Verification items for the finished model (mm, model axes). A direction names the side the tool comes from. Round coordinates to 2 decimals unless told otherwise and drop trailing zeros. Order: outer loops, then holes, each group sorted by start corner. A loop starts at its lowest first (then second) coordinate and runs counter-clockwise, first axis right, second up. Notation, with made-up numbers: (46, 25) -> (59, 25) arc R14 cw to (59, 42) -> close; hole circle Ø11 at (8, 17). An arc over 180 degrees is marked (long way). Return JSON: item names as keys, results as strings. Group by question number.
1) Tool access check on faces 1 (the cylindrical face through (0.867, -3.905, 0.159)), 2 (the cylindrical face through (4.619, -1.915, 13.795)). Record the directions out of +Z, -Z, +X, -X, +Y, -Y that give a thin tool (end or side, any length) a straight path to the whole face; none if there is none.
2) Section check A-A on z = 70.5. Enter the section's corners in (x, y), plus the area to 3 significant figures.
3) Depth check by flat-ended pin: pin 1 (2 mm diameter, centred on y = 3.5, z = 51.5, fed in from -X); pin 2 (5 mm diameter, centred on x = -3, z = 58, fed in from +Y); pin 3 (6 mm diameter, centred on y = -3.5, z = 72, fed in from +X). Enter the tip coordinate at first touch or a pass-through.
4) Draft check along Z on faces 3 (the cylindrical face through (4.619, -1.915, 46.394)), 4 (the cylindrical face through (0.867, -3.905, 27.893)), 5 (the flat face through (0, 0, 135)). Enter one of: pulls with the +Z half, pulls with the -Z half, needs draft (parallel to the pull), parting line crosses it, or undercut.
5) Scan lines: L1, parallel to Z at x = 4, y = -2.25 (3 decimals); L2, parallel to X at y = -0.5, z = 119; L3, parallel to Y at x = 0.25, z = 42. Record each from-to range of solid material in increasing order.
```python
from build123d import *

# Parameters (mm, degrees)
SKETCH1_R           = 5
BOSS_EXTRUDE1_DEPTH = 135
SKETCH2_W           = 1
SKETCH2_H           = 0.8
BOSS_EXTRUDE2_START = 5
SKETCH3_R           = 5
BOSS_EXTRUDE2_DEPTH = 5
SKETCH4_R           = 5
SKETCH4_R_2         = 4
CUT_EXTRUDE1_DEPTH  = 0.8
SKETCH5_R           = 5
SKETCH5_R_2         = 4
CUT_EXTRUDE2_DEPTH  = 1


with BuildPart() as part:
    # Sketch1 → Boss-Extrude1 (new body)
    with BuildSketch(Plane.XY):
        Circle(SKETCH1_R)
    extrude(amount=BOSS_EXTRUDE1_DEPTH)

    # Sketch2 → Cut-Revolve1 (revolve, cut)
    with BuildSketch(Plane(origin=(0, 0, 0), x_dir=(1, 0, 0), z_dir=(0, 1, 0))):
        with Locations((-4.5, -65.3)):
            Rectangle(SKETCH2_W, SKETCH2_H)
        with Locations((-4.5, -93.4)):
            Rectangle(SKETCH2_W, SKETCH2_H)
    revolve(axis=Axis((0, 0, 6.050553304), (0, 0, 1)), mode=Mode.SUBTRACT)

    # Sketch3 → Boss-Extrude2 (add)
    with BuildSketch(Plane(origin=(0, 0, 0), x_dir=(-1, 0, 0), z_dir=(0, 0, -1)).offset(BOSS_EXTRUDE2_START)):
        Circle(SKETCH3_R)
    extrude(amount=-BOSS_EXTRUDE2_DEPTH)

    # Sketch4 → Cut-Extrude1 (cut)
    with BuildSketch(Plane(origin=(-672.545878218, -100.484437541, -0.235), x_dir=(-0.3247374432468007, 0.945804204343336, 0), z_dir=(0, 0, -1))):
        with Locations(Location((-123.362225461, 668.727778566, 0), (0, 0, 288.949668831))):
            Circle(SKETCH4_R)
        with Locations(Location((-123.362225461, 668.727778566, 0), (0, 0, 288.949668831))):
            Circle(SKETCH4_R_2, mode=Mode.SUBTRACT)
    extrude(amount=-CUT_EXTRUDE1_DEPTH, mode=Mode.SUBTRACT)

    # Sketch5 → Cut-Extrude2 (cut)
    with BuildSketch(Plane(origin=(-672.545878218, -100.484437541, 27.4), x_dir=(-0.3247374432468007, 0.945804204343336, 0), z_dir=(0, 0, -1))):
        with Locations(Location((-123.362225461, 668.727778566, 0), (0, 0, 288.949668831))):
            Circle(SKETCH5_R)
        with Locations(Location((-123.362225461, 668.727778566, 0), (0, 0, 288.949668831))):
            Circle(SKETCH5_R_2, mode=Mode.SUBTRACT)
    extrude(amount=-CUT_EXTRUDE2_DEPTH, mode=Mode.SUBTRACT)


solid = part.part
```
Check result:
{
 "1": {"face 1": "none", "face 2": "+Z, -Z"},
 "2": {"outline": "circle Ø10 at (0, 0)", "area": "78.5 mm^2"},
 "3": {"pin 1": "x = -4.33", "pin 2": "y = 4.97", "pin 3": "x = 4.97"},
 "4": {"face 3": "needs draft", "face 4": "undercut", "face 5": "pulls with the +Z half"},
 "5": {"L1": "-5 to -0.235, 0.565 to 27.4, 28.4 to 64.9, 65.7 to 93, 93.8 to 135", "L2": "-4.97 to 4.97", "L3": "-4.99 to 4.99"}
}
